For this review, use the dimensioned drawing (mm, ordinates from the lowest corner) and the shaded views. A direction names the side the tool comes from. Coordinates: 2 decimals unless noted, no trailing zeros. Write each loop counter-clockwise with the first axis right and the second up, starting at its lowest first coordinate (ties: lowest second). Pieces come first, ordered by that corner, then holes. Notation, with made-up numbers: (41, 85.25) - (61, 85.25) arc R21 cw to (61, 91.25) - close; hole circle Ø8 at (52.5, -23.5). An arc over 180 degrees is marked (long way). One line per item, written item: value.
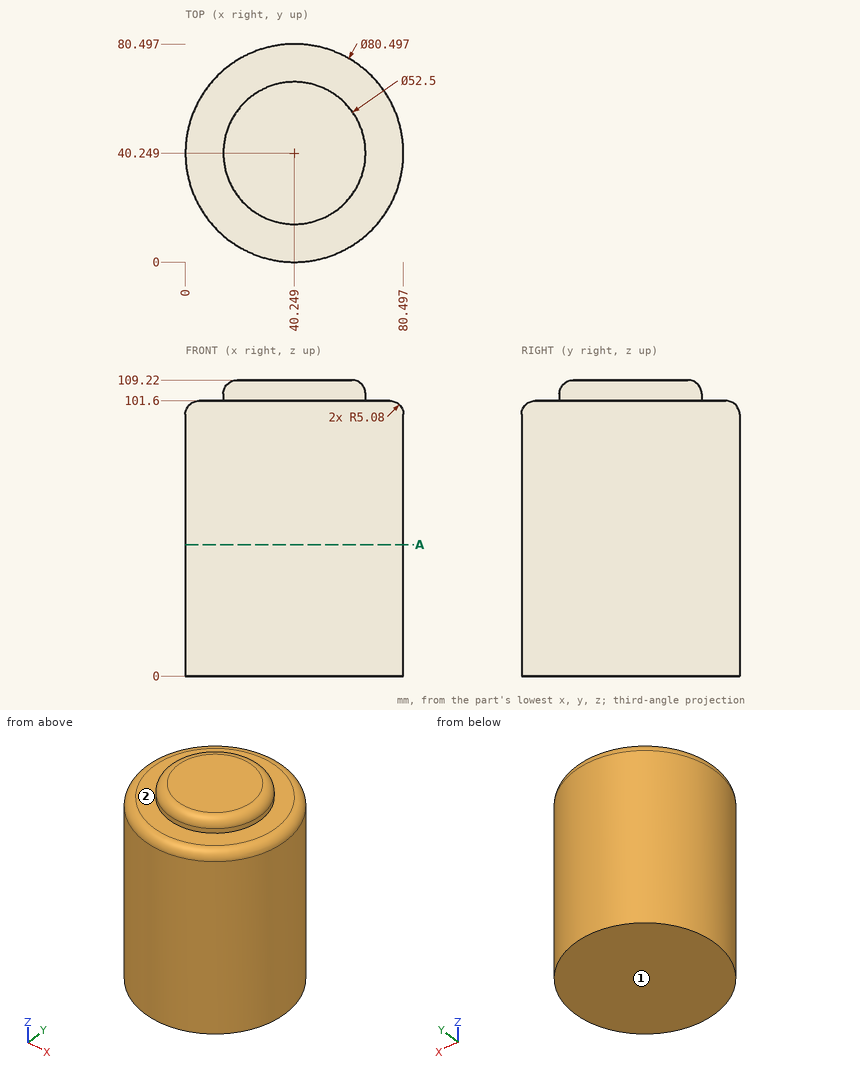
1. Consider section A-A, the plane z = 48.5. Write out the cut boundary in (x, y).
Answer block:
outline: circle Ø80.5 at (40.25, 40.25)
2. For the marked faces 1 and 2, list the 3-axis set-ups (+Z, -Z, +X, -X, +Y, -Y) from which the entire face can be reached by the end or side of a thin tool; tool diameter is ignored.
Answer block:
face 1: -Z, +X, -X, +Y, -Y
face 2: +Z
3. Wall thickness on line 1 along X through (y, z) = (39, 7); line 2 along Z through (x, y) = (20.5, 68); line 3 along Y through (x, z) = (25.5, 66): over which ranges is each line inside the solid? List them lowest first.
Answer block:
line 1: x = 0.02 to 80.48
line 2: z = 0 to 101.6
line 3: y = 2.8 to 77.7
4. Insertion check: pin 1 Ø10 at (y, z) = (43.5, 41) entering from -X; pin 2 Ø3 at (y, z) = (48.5, 11.5) entering from -X; pin 3 Ø8 at (x, y) = (68.5, 70.5) entering from +Z; pin 4 Ø1 at (x, z) = (12, 90.5) entering from +Y. Each pin has a flat end and moves straight along its axis. Give the tip position at first contact, or say it passes through.
Answer block:
pin 1: stops at x = 0
pin 2: stops at x = 0.57
pin 3: stops at z = 101.09
pin 4: stops at y = 69.4
